Work out the finished part from the listing and answer in its coordinate system (mm). A direction names the side the tool comes from. Give positions to 0.01 mm unless a question says otherwise; leave off trailing zeros. Order: outer loops, then holes, each group sorted by start corner. A loop starts at its lowest first (then second) coordinate and runs counter-clockwise, first axis right, second up. Notation, with made-up numbers: (-13, -22.75) - (41, -22.75) arc R21 ccw to (41, 10.25) - close; hole circle Ø11 at (-31.75, -11). An arc over 180 degrees is marked (long way). Put each result on its own line as item: value.
```python
from build123d import *

# Parameters (mm, degrees)
EXTRUDE_THIN1_DEPTH = 203.2
SKETCH2_W           = 711.2
SKETCH2_H           = 312.7375
BOSS_EXTRUDE1_DEPTH = 1.5875


with BuildPart() as part:
    # Sketch1 → Extrude-Thin1 (new body, symmetric)
    with BuildSketch(Plane(origin=(0, 0, 0), x_dir=(0, 0, -1), z_dir=(1, 0, 0))):
        with BuildLine():
            ThreePointArc((60.57513929, -138.1125), (126.253511536, -82.489156748), (150.8125, 0))
            Line((150.8125, 0), (150.8125, 312.7375))
            Line((150.8125, 312.7375), (152.4127, 312.7375))
            Line((152.4127, 312.7375), (152.4127, 0))
            ThreePointArc((152.4127, 0), (127.593127743, -83.364410117), (61.217873399, -139.577946316))
            Line((61.217873399, -139.577946316), (60.57513929, -138.1125))
        make_face()
    extrude(amount=EXTRUDE_THIN1_DEPTH, both=True)

    # Sketch2 → Boss-Extrude1 (add)
    with BuildSketch(Plane.XY.offset(-150.8125)):
        with Locations((0, 156.36875)):
            Rectangle(SKETCH2_W, SKETCH2_H)
    extrude(amount=-BOSS_EXTRUDE1_DEPTH)


solid = part.part
```
(1) Section D-D, the plane x = -283.5 is taken. Write down the section's boundary in (y, z), then the cut area to 3 significant figures.
Geometry check:
outline: (0, -152.4) - (312.74, -152.4) - (312.74, -150.81) - (0, -150.81) - close
area: 496 mm²
(2) Section C-C, the plane z = -128 is taken. Write down the section's boundary in (x, y), then the cut area to 3 significant figures.
Geometry check:
outline: (-203.2, -82.74) - (203.2, -82.74) - (203.2, -79.75) - (-203.2, -79.75) - close
area: 1,210 mm²
(3) Section A-A, the plane x = -5.5 is taken. Write down the section's boundary in (y, z) (1 decimal).
Geometry check:
outline: (-139.6, -61.2) arc R152.4 ccw to (0, -152.4) - (312.7, -152.4) - (312.7, -150.8) - (0, -150.8) arc R150.8 cw to (-138.1, -60.6) - close
(4) Given pin 1 (1.7 mm diameter, centred on x = -287, z = -151.5, fed in from -Y); pin 2 (2 mm diameter, centred on x = 204, z = -73.5, fed in from -Y); pin 3 (5 mm diameter, centred on x = 201, y = -22, fed in from +Z), each flat-ended and moving along its own axis, determine where each tip first touches the part or whether it passes through.
Geometry check:
pin 1: stops at y = 0
pin 2: stops at y = -133.85
pin 3: stops at z = -148.81
(5) A tool of negligible diameter and unlimited length cuts with its end or side. For faces 1 (the face through (2.845, -82.328, -128.264)), 2 (the face through (-5, 159, -150.812)), from which of +Z, -Z, +X, -X, +Y, -Y can it reach the whole face along a straight path? Write none if from no direction.
Geometry check:
face 1: -Z, +X, -X, -Y
face 2: +Z, +X, -X, +Y
(6) Straight lines are drawn through the part: line 1 (Z direction, x = -19, y = 73); line 2 (Y direction, x = 93.5, z = -94.5); line 3 (Y direction, x = -33, z = -78). For each, find the intervals that lie inside material, in ascending order.
Geometry check:
line 1: z = -152.41 to -150.81
line 2: y = -119.58 to -117.53
line 3: y = -130.94 to -129.08
